Geometry check sheet. Reference: the model listing, model coordinates, mm. A direction names the side the tool comes from. Coordinates: 2 decimals unless noted, no trailing zeros. Order: outer loops, then holes, each group sorted by start corner. A loop starts at its lowest first (then second) coordinate and runs counter-clockwise, first axis right, second up.
```python
from build123d import *

# Parameters (mm, degrees)
BOSS_EXTRUDE1_DEPTH     = 290
CUT_EXTRUDE1_DEPTH      = 290
CUT_EXTRUDE1_DEPTH_BACK = 290
SHELL3_T                = -1.5
SKETCH3_R               = 2.5
CUT_EXTRUDE2_DEPTH      = 20
SKETCH4_R               = 2.5
CUT_EXTRUDE3_DEPTH      = 18
CUT_EXTRUDE4_DEPTH      = 119
CUT_EXTRUDE4_DEPTH_BACK = 128


with BuildPart() as part:
    # Sketch1 → Boss-Extrude1 (new body)
    with BuildSketch(Plane.XY):
        with BuildLine():
            Line((-4, -11.842719282), (-204, -120.795710387))
            Line((-204, -120.795710387), (-204, 120.795710387))
            Line((-204, 120.795710387), (-4, 11.842719282))
            Line((-4, 11.842719282), (-4, 8.61684397))
            ThreePointArc((-4, 8.61684397), (-9.5, 0), (-4, -8.61684397))
            Line((-4, -8.61684397), (-4, -11.842719282))
        make_face()
    extrude(amount=BOSS_EXTRUDE1_DEPTH)

    # Sketch2 → Cut-Extrude1 (cut, two sides: drawn at the far end of the back side and taken through both)
    with BuildSketch(Plane(origin=(0, 0, 0), x_dir=(-1, 0, 0), z_dir=(0, -1, 0)).offset(-CUT_EXTRUDE1_DEPTH_BACK)):
        Polygon((4, -189), (204, -290), (4, -290), align=None)
        Polygon((4, -101), (204, 0), (4, 0), align=None)
    extrude(amount=CUT_EXTRUDE1_DEPTH + CUT_EXTRUDE1_DEPTH_BACK, mode=Mode.SUBTRACT)

    # Shell3
    shell3_openings = [part.faces().sort_by_distance(p)[0] for p in [
        (-204, 0, 145),
        (-9.5, 0, 145),
    ]]
    offset(amount=SHELL3_T, openings=shell3_openings, kind=Kind.INTERSECTION)

    # Sketch3 → Cut-Extrude2 (cut)
    with BuildSketch(Plane(origin=(4.059646396, -7.452106372, 0), x_dir=(-0.8781500169152763, -0.47838535490930323, 0), z_dir=(0.4783853549093033, -0.8781500169152764, 0))):
        with Locations(Location((21.727983535, -175, 0), (0, 0, 180))):
            Circle(SKETCH3_R)
        with Locations(Location((21.727983535, -115, 0), (0, 0, 180))):
            Circle(SKETCH3_R)
    extrude(amount=-CUT_EXTRUDE2_DEPTH, mode=Mode.SUBTRACT)

    # Sketch4 → Cut-Extrude3 (cut)
    with BuildSketch(Plane(origin=(4.059646396, 7.452106372, 0), x_dir=(0.8781500169152766, -0.47838535490930256, 0), z_dir=(0.47838535490930256, 0.8781500169152766, 0))):
        with Locations(Location((-21.727983535, -115, 0), (0, 0, 180))):
            Circle(SKETCH4_R)
        with Locations(Location((-21.727983535, -175, 0), (0, 0, 180))):
            Circle(SKETCH4_R)
    extrude(amount=-CUT_EXTRUDE3_DEPTH, mode=Mode.SUBTRACT)

    # Sketch6 → Cut-Extrude4 (cut, two sides: drawn at the far end of the back side and taken through both)
    with BuildSketch(Plane.XY.offset(145).offset(-CUT_EXTRUDE4_DEPTH_BACK)):
        with BuildLine():
            Line((-4, 11.842719282), (-4, -11.842719282))
            ThreePointArc((-4, -11.842719282), (-12.5, 0), (-4, 11.842719282))
        make_face()
    extrude(amount=CUT_EXTRUDE4_DEPTH + CUT_EXTRUDE4_DEPTH_BACK, mode=Mode.SUBTRACT)


solid = part.part
```
Item 1: Depth check by flat-ended pin: P1, Ø10, axis at y = 71, z = 154.5, coming from the +X side; P2, Ø4, axis at x = -176.5, z = 94.5, coming from the -Y side; P3, Ø4, axis at y = -59, z = 56, coming from the -X side. Enter the tip coordinate at first touch or a pass-through.
Item 2: Sectioned sample at C-C (y = -91). Record the cut outline in (x, z), and give its area (3 significant figures).
Item 3: Tool access check on faces 4 (the face through (-127.622, 79.188, 142.97)), 5 (the face through (-125.519, 1.667, 41.313)). Record the directions out of +Z, -Z, +X, -X, +Y, -Y that give a thin tool (end or side, any length) a straight path to the whole face; none if there is none.
Item 4: Sectioned sample at A-A (z = 158.5). Record the cut outline in (x, y).
Item 5: Sectioned sample at B-B (x = -131). Record the cut outline in (y, z) (3 decimals), and give its area (3 significant figures).
Item 6: Release check for a two-part mould opening along Z. For faces 1 (the face through (-124.82, -77.66, 142.97)), 2 (the face through (-125.519, -76.334, 142.994)), 3 (the face through (-124.822, 1.691, 250.015)) record: pulls with the +Z half, pulls with the -Z half, needs draft (parallel to the pull), parting line crosses it, or undercut.
Item 7: Sectioned sample at D-D (z = 83.5). Record the cut outline in (x, y).
Item 8: Thickness scan on line 1 along Y through (x, z) = (-71, 212); line 2 along Y through (x, z) = (-192.5, 41.5); line 3 along Z through (x, y) = (-67, -6) (3 decimals). Record the ranges inside material, lowest first.
Geometry check:
1. P1: stops at x = -103.41
1. P2: stops at y = -106.9
1. P3: stops at x = -100.4
2. outline: (-204, 0) - (-149.31, 27.62) - (-149.31, 262.38) - (-204, 290) - (-204, 288.32) - (-152.44, 262.28) - (-152.44, 27.72) - (-204, 1.68) - close
2. area: 914 mm2
3. face 4: +Z, -Z, +X, +Y
3. face 5: -X
4. outline: (-204, -120.8) - (-4, -11.84) arc R12.5 cw to (-5.76, -11.09) - (-204, -119.09) - close; (-204, 119.09) - (-5.76, 11.09) arc R12.5 cw to (-4, 11.84) - (-204, 120.8) - close
5. outline: (-81.028, 36.865) - (81.028, 36.865) - (81.028, 253.135) - (-81.028, 253.135) - close; hole (-79.32, 38.545) - (79.32, 38.545) - (79.32, 251.455) - (-79.32, 251.455) - close
5. area: 1,270 mm2
6. face 1: needs draft
6. face 2: undercut
6. face 3: pulls with the +Z half
7. outline: (-204, -120.8) - (-38.65, -30.72) - (-38.65, 30.72) - (-204, 120.8) - (-204, 119.09) - (-41.98, 30.83) - (-41.98, -30.83) - (-204, -119.09) - close
8. line 1: y = -48.34 to -46.63, 46.63 to 48.34
8. line 2: y = -114.53 to -112.82, 112.82 to 114.53
8. line 3: z = 69.185 to 70.865, 219.135 to 220.815
